Study the drawing (mm; zero at the part's minimum x, y, z) and answer. A direction names the side the tool comes from. Coordinates: 2 decimals unless noted, no trailing zeros. Order: outer loops, then holes, each group sorted by start corner. A loop starts at its lowest first (then second) coordinate and runs counter-clockwise, first axis right, second up. Notation, with made-up numbers: (46, -31) -> (100, -31) arc R27 cw to (100, -11) -> close; hole circle Ø11 at (82.5, 10.5). An arc over 180 degrees is marked (long way). Answer in a Markdown table with one row per item. Add a question column.
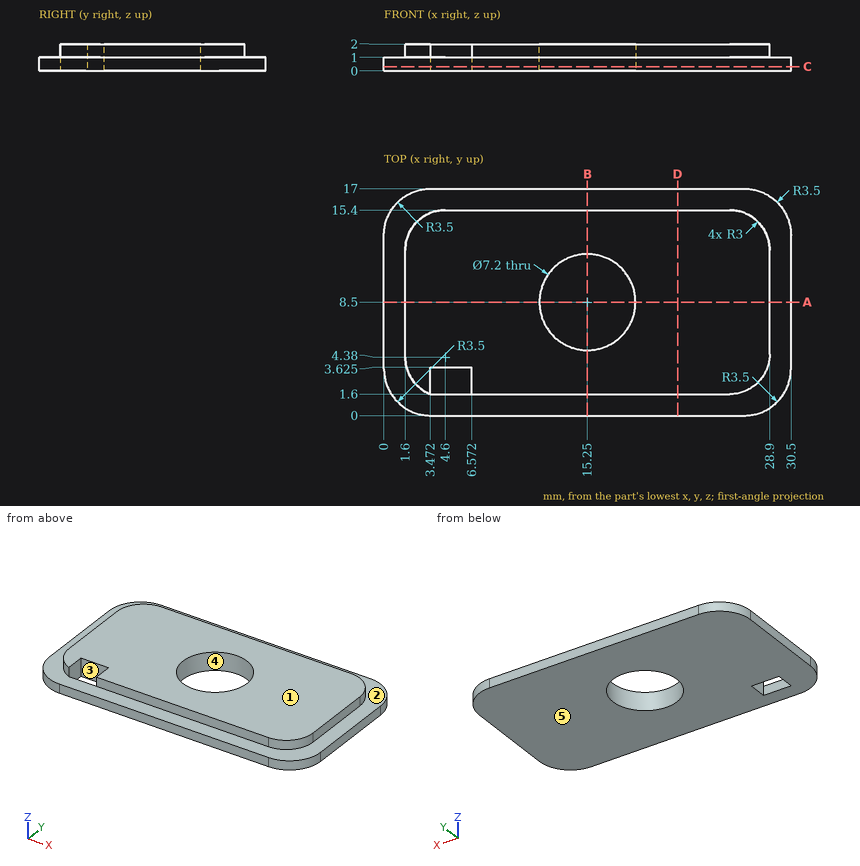
Q1. A cutting plane is placed at D-D (x = 22). Determine the outline of the cut face in (y, z), then the cut area to 3 significant figures.
Q2. A cutting plane is placed at B-B (x = 15.25). Determine the outline of the cut face in (y, z), then the cut area to 3 significant figures.
Q3. Straight lines are drawn through the part: line 1 (Y direction, x = 15.25, z = 1.05); line 2 (Y direction, x = 8, z = 1.4); line 3 (X direction, y = 3.5, z = 1.1). For each, find the intervals that lie inside material, in ascending order.
Q4. A cutting plane is placed at C-C (z = 0.3). Determine the outline of the cut face in (x, y) (3 decimals), then the cut area to 3 significant figures.
Q5. Determine the mould class of the marked faces 3, 4 and 5 for opening direction X: +X half, -X half, draft (parallel to the pull), parting line (faces both ways), or undercut.
Q6. For the marked faces 1 and 2, determine the directions among +Z, -Z, +X, -X, +Y, -Y from which every point of the face is accessible in a straight line to the end or side of a thin tool.
Q7. A cutting plane is placed at A-A (y = 8.5). Determine the outline of the cut face in (x, z).
Q8. Given pin 1 (0.5 mm diameter, centred on x = 20, z = 1.5, fed in from -Y); pin 2 (0.5 mm diameter, centred on y = 8.5, z = 1.5, fed in from -X), each flat-ended and moving along its own axis, determine where each tip first touches the part or whether it passes through.
Returned:
| question | item | result |
|---|---|---|
| 1 | outline | (0, 0) -> (17, 0) -> (17, 1) -> (15.4, 1) -> (15.4, 2) -> (1.6, 2) -> (1.6, 1) -> (0, 1) -> close |
| 1 | area | 30.8 mm² |
| 2 | outline | (0, 0) -> (4.9, 0) -> (4.9, 2) -> (1.6, 2) -> (1.6, 1) -> (0, 1) -> close; (12.1, 0) -> (17, 0) -> (17, 1) -> (15.4, 1) -> (15.4, 2) -> (12.1, 2) -> close |
| 2 | area | 16.4 mm² |
| 3 | line 1 | y = 1.6 to 4.9, 12.1 to 15.4 |
| 3 | line 2 | y = 1.6 to 15.4 |
| 3 | line 3 | x = 1.73 to 3.47, 6.57 to 28.69 |
| 4 | outline | (0, 3.5) arc R3.5 ccw to (3.5, 0) -> (27, 0) arc R3.5 ccw to (30.5, 3.5) -> (30.5, 13.5) arc R3.5 ccw to (27, 17) -> (3.5, 17) arc R3.5 ccw to (0, 13.5) -> close; hole (3.472, 1.6) -> (6.572, 1.6) -> (6.572, 3.625) -> (3.472, 3.625) -> close; hole circle Ø7.2 at (15.25, 8.5) |
| 4 | area | 461 mm² |
| 5 | face 3 | undercut |
| 5 | face 4 | undercut |
| 5 | face 5 | draft |
| 6 | face 1 | +Z, +X, -X, +Y, -Y |
| 6 | face 2 | +Z |
| 7 | outline | (0, 0) -> (11.65, 0) -> (11.65, 2) -> (1.6, 2) -> (1.6, 1) -> (0, 1) -> close; (18.85, 0) -> (30.5, 0) -> (30.5, 1) -> (28.9, 1) -> (28.9, 2) -> (18.85, 2) -> close |
| 8 | pin 1 | stops at y = 1.6 |
| 8 | pin 2 | stops at x = 1.6 |
